Verification items for the finished model (mm, model axes). Coordinates: 2 decimals unless noted, no trailing zeros. Loops run counter-clockwise (first coordinate to the right, second up) from the corner with the lowest first, then second, coordinate; pieces in that order, holes last. Notation, with made-up numbers: (39.5, 32.5) -> (83.5, 32.5) arc R15 cw to (83.5, 44.5) -> close; hole circle Ø4 at (-29, -11). An arc over 180 degrees is marked (long way). Write item = value, one per line.
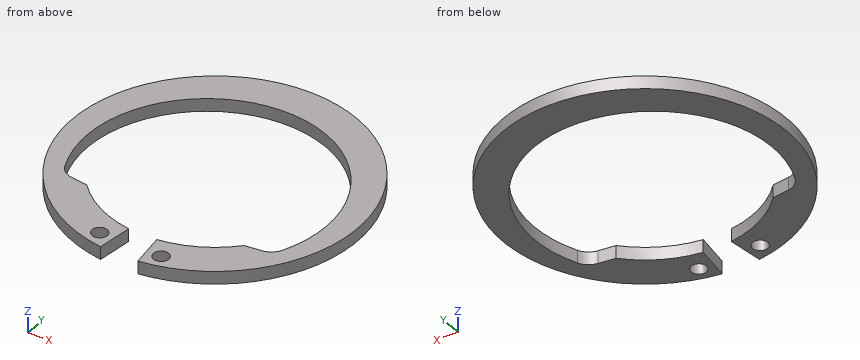
```python
from build123d import *

# Parameters (mm, degrees)
BODYSKE_R  = 0.5334
BODY_DEPTH = 0.889


with BuildPart() as part:
    # BodySke → Body (new body)
    with BuildSketch(Plane.XY):
        with BuildLine():
            Line((-0.974717393, -7.403713647), (-1.29299246, -9.821252797))
            ThreePointArc((-1.29299246, -9.821252797), (0, 9.906), (1.29299246, -9.821252797))
            Line((1.29299246, -9.821252797), (0.974717393, -7.403713647))
            ThreePointArc((0.974717393, -7.403713647), (3.420903654, -6.63795661), (5.464040708, -5.090118751))
            Line((5.464040708, -5.090118751), (6.625562126, -4.937201555))
            ThreePointArc((6.625562126, -4.937201555), (7.192072795, -4.707317059), (7.574660301, -4.230443889))
            ThreePointArc((7.574660301, -4.230443889), (0, 7.4676), (-7.574660301, -4.230443889))
            ThreePointArc((-7.574660301, -4.230443889), (-7.192072795, -4.707317059), (-6.625562126, -4.937201555))
            Line((-6.625562126, -4.937201555), (-5.464040708, -5.090118751))
            ThreePointArc((-5.464040708, -5.090118751), (-3.420903654, -6.63795661), (-0.974717393, -7.403713647))
        make_face()
        with Locations((2.133243521, -8.662961107)):
            Circle(BODYSKE_R, mode=Mode.SUBTRACT)
        with Locations((-2.133243521, -8.662961107)):
            Circle(BODYSKE_R, mode=Mode.SUBTRACT)
    extrude(amount=-BODY_DEPTH)


solid = part.part
```
1) Material ranges on line 1 (Y direction, x = -2.5, z = -0.6); line 2 (Y direction, x = -1.75, z = -0.7); line 3 (Y direction, x = 0, z = -0.25), recorded low to high.
Ans:
line_1 = -9.59 to -9.05, -8.28 to -7.04, 7.08 to 9.59
line_2 = -9.75 to -9.03, -8.29 to -7.26, 7.28 to 9.75
line_3 = 7.47 to 9.91
2) Sectioned sample at C-C, the plane z = -0.2. Record the cut outline in (x, y).
Ans:
outline = (-7.57, -4.23) arc R8.3 cw (long way) to (7.57, -4.23) arc R1.21 cw to (6.63, -4.94) -> (5.46, -5.09) arc R7.47 cw to (0.97, -7.4) -> (1.29, -9.82) arc R9.91 ccw (long way) to (-1.29, -9.82) -> (-0.97, -7.4) arc R7.47 cw to (-5.46, -5.09) -> (-6.63, -4.94) arc R1.21 cw to start; hole circle Ø1.07 at (-2.13, -8.66); hole circle Ø1.07 at (2.13, -8.66)
3) Sectioned sample at D-D, the plane x = 0. Record the cut outline in (y, z).
Ans:
outline = (7.47, -0.89) -> (9.91, -0.89) -> (9.91, 0) -> (7.47, 0) -> close
4) Sectioned sample at A-A, the plane x = -4.5. Record the cut outline in (y, z).
Ans:
outline = (-8.82, -0.89) -> (-5.96, -0.89) -> (-5.96, 0) -> (-8.82, 0) -> close; (6.14, -0.89) -> (8.82, -0.89) -> (8.82, 0) -> (6.14, 0) -> close
5) Depth check by flat-ended pin: pin 1 Ø1.2 at (x, y) = (-2.13, -8.66) entering from +Z; pin 2 Ø0.9 at (x, y) = (2.13, -8.66) entering from -Z. Enter the tip coordinate at first touch or a pass-through.
Ans:
pin_1 = 0
pin_2 = through
6) Sectioned sample at B-B, the plane y = 6.5. Record the cut outline in (x, z).
Ans:
outline = (-7.48, -0.89) -> (-3.89, -0.89) -> (-3.89, 0) -> (-7.48, 0) -> close; (3.89, -0.89) -> (7.48, -0.89) -> (7.48, 0) -> (3.89, 0) -> close
